Autodesk Inventor part; units mm, degrees
ref_plane "Work Plane3" through (14, 0, 0) normal (-1, 0, 0) x (0, 0, 1)
ref_plane "YZ Plane" through (0, 0, 0) normal (1, 0, 0) x (0, 1, 0)
ref_plane "XZ Plane" through (0, 0, 0) normal (0, 1, 0) x (-1, 0, 0)
sketch "Sketch1" plane through (0, 0, 0) normal (0, 0, 1) x (1, 0, 0)
  line L0 (0, 0) -> (28, 0)
  line L1 (28, 0) -> (28, 28)
  line L2 (28, 28) -> (0, 28)
  line L3 (0, 28) -> (0, 0)
  circle A0 centre (7, 0) radius 4
  circle A1 centre (21, 0) radius 4
  point P0 (3, 0)
  point P1 (11, 0)
  point P2 (17, 0)
  point P3 (25, 0)
  dimension "d0" = 28
  dimension "d1" = 28
  dimension "d2" = 8
  dimension "d3" = 8
  dimension "d4" = 14
  dimension "d5" = 7
  dimension "d6" = 7
extrude "Extrusion1" add sketch "Sketch1" along normal blind 12 contours A1 L0 A0 L3 L2 L1
chamfer "Chamfer1" distance 0.5 angle 45 4 edges at (3, 0, 6) (11, 0, 6) (17, 0, 6) (25, 0, 6)
sketch "Sketch2" plane through (0, 28, 0) normal (0, 1, 0) x (1, 0, 0)
  circle A0 centre (14, -6) radius 6.35
  line L0 (28, 0) -> (0, 0)
  line L1 (28, 0) -> (28, -12)
  point P0 (14, 0)
  point P1 (28, -6)
  point P2 (16.0791, 0)
  point P3 (11.9209, 0)
  dimension "d12" = 12.7
extrude "Extrusion2" cut sketch "Sketch2" against normal blind 4 contours A0 L0 picked at (13.6383, -8.0675)
fillet "Fillet1" radius 0.25 4 edges at (11.9209, 26, 0) (16.0791, 26, 0) (11.9209, 26, 12) (16.0791, 26, 12)
ref_plane "Work Plane3" through (14, 0, 0) normal (-1, 0, 0) x (0, 0, 1)
sketch "Sketch5" plane through (0, 0, 0) normal (0, -1, 0) x (1, 0, 0)
  circle A0 centre (-3.5, 6) radius 2
  circle A1 centre (-3.5, 6) radius 3.5
  circle A2 centre (-3.5, 6) radius 6
  line L0 (2.5, 12) -> (2.5, 0)
  line L1 (0, 12) -> (2.5, 12)
  line L2 (0, 0) -> (0, 12)
  line L3 (0, 0) -> (2.5, 0)
  line L4 (0, 0) -> (0, 12)
  line L5 (0, 0) -> (-5.9853, 0)
  line L6 (-5.9853, 0) -> (-7.7426, 1.7574)
  line L7 (0, 12) -> (-5.9853, 12)
  line L8 (-5.9853, 12) -> (-7.7426, 10.2426)
  line L9 (0, 0) -> (0, 12)
  dimension "d22" = 4
  dimension "d23" = 7
  dimension "d24" = 135
  dimension "d25" = 135
extrude "Extrusion3" add sketch "Sketch5" against normal blind 7 contours A0 | A1 | L2 A2 | L2 L5 A2 | A2 L7 L2 | L5 L6 A2 | A2 L8 L7 picked at (-7.4809, 9.2519)
sketch "Sketch6" plane through (2.5, 0, 0) normal (0, -1, 0) x (1, 0, 0)
  arc A0 (-10.2426, 10.2426) -> (-10.2426, 1.7574) centre (-6, 6) ccw
  point P0 (-2.5, 0)
hole "Hole1" at (-3.5, 0, 6) direction (0, 1, 0) diameter 4 end through all
mirror "Mirror2" about plane through (14, 0, 0) normal (-1, 0, 0) of "Extrusion3", "Hole1"
sketch "Sketch7" plane through (0, 0, 12) normal (0, 0, 1) x (1, 0, 0)
  line L0 (17.24, 24) -> (10.76, 24)
  line L1 (17.1173, 24) -> (17.24, 24)
  line L2 (17.1173, 24) -> (17.1173, 24)
  line L3 (17.24, 24) -> (17.1173, 24)
  line L4 (10.76, 24) -> (17.24, 24)
  line L5 (10.8827, 24) -> (10.76, 24)
  line L6 (10.8827, 24) -> (10.8827, 24)
  line L7 (10.76, 24) -> (10.8827, 24)
  line L8 (17.1173, 24) -> (20.35, 24)
  line L9 (7.65, 24) -> (10.8827, 24)
  line L10 (28, 28) -> (17.24, 28)
  line L11 (22.62, 28) -> (22.62, 24)
  line L12 (28, 7) -> (28, 28)
  line L13 (22.62, 24) -> (28, 7)
  line L14 (10.76, 28) -> (0, 28)
  line L15 (5.38, 28) -> (5.38, 24)
  line L16 (0, 28) -> (0, 7)
  line L17 (5.38, 24) -> (0, 7)
  line L18 (17.24, 24) -> (10.76, 24)
  point P0 (0, 0)
extrude "Extrusion4" cut sketch "Sketch7" against normal through all
chamfer "Chamfer2" distance 2 angle 45 8 edges at (22.62, 26, 12) (25.31, 15.5, 12) (22.62, 26, 0) (25.31, 15.5, 0) (2.69, 15.5, 12) (2.69, 15.5, 0) (5.38, 26, 0) (5.38, 26, 12)
equation "\"d1\" = MotorHeight"
equation "\"d5\" = d6"
equation "\"MotorHeight\" = MotorHeightBase"
properties part number "Magnet Mount"
Can you work these out from the model? Positions are in its coordinate system, mm. A direction names the side the tool comes from. Coordinates: 2 decimals unless noted, no trailing zeros. Order: outer loops, then holes, each group sorted by start corner. A loop starts at its lowest first (then second) coordinate and runs counter-clockwise, first axis right, second up. Notation, with made-up numbers: (-37, 75.5) - (1, 75.5) arc R19 ccw to (1, 111.5) - close; hole circle Ø1 at (29.25, 0.25). An arc over 180 degrees is marked (long way). Answer as a JSON object with one key per item and string values. Group by question number.
Q1. Imagine slicing it at B-B (z = 6). Give the number of separate pieces and of enclosed holes in the cut face, and give its area (3 significant figures).
Q2. We'd pull the mould along X, two halves only. Please class faces 1 (the face through (-1, 0, 6)), 2 (the face through (24.258, 15.462, 11.014)), 3 (the face through (7.65, 26.03, 5.91)): +X half, -X half, draft (parallel to the pull), parting line (faces both ways), or undercut.
Q3. Imagine slicing it at D-D (x = 15). Please give me the cut outline in (y, z), and give its area (3 significant figures).
Q4. On a 3-axis mill with a long thin cutter (end or side, diameter ignored), from which of +Z, -Z, +X, -X, +Y, -Y can I reach the whole of each face in a straight line? I mean faces 4 (the face through (6.39, 25.88, 11.01)), 5 (the face through (21.63, 25.82, 1.01)), 6 (the face through (14, 24, 6)), 7 (the face through (22.62, 26, 6)). Say none if no direction works.
Q5. Imagine slicing it at C-C (y = 13.75). Please give me the cut outline in (x, z).
Q6. Imagine slicing it at A-A (x = -3.5). Please give me the cut outline in (y, z), and give its area (3 significant figures).
Q7. I need wall thicknesses on line 1 (X direction, y = 4.25, z = 6); line 2 (X direction, y = 3.5, z = 9.5); line 3 (Z direction, x = 31.5, y = 2). Which ranges of each line are inside material? Lowest first, please. Write a range as from..to.
Q8. Will these pins go through, and if not, where does the flat tip stop? P1, Ø1, axis at x = 12.5, z = 2, coming from the -Y side; P2, Ø1, axis at x = 17.5, z = 5.5, coming from the -Y side; P3, Ø2.5, axis at x = 31.5, z = 6, coming from the +Y side; P4, Ø4, axis at y = 15, z = 8, coming from the +X side.
Determined:
{
 "1": {"separate pieces": "3", "enclosed holes": "0", "area": "625 mm2"},
 "2": {"face 1": "draft", "face 2": "+X half", "face 3": "undercut"},
 "3": {"outline": "(0, 0) - (24, 0) - (24, 12) - (0, 12) - close", "area": "288 mm2"},
 "4": {"face 4": "+Z, -X, +Y", "face 5": "-Z, +X, +Y", "face 6": "+Y", "face 7": "+Z, -Z, +X, +Y"},
 "5": {"outline": "(2.14, 2) - (4.23, 0) - (23.77, 0) - (25.86, 2) - (25.86, 10) - (23.77, 12) - (4.23, 12) - (2.14, 10) - close"},
 "6": {"outline": "(0, 0) - (7, 0) - (7, 4) - (0, 4) - close; (0, 8) - (7, 8) - (7, 12) - (0, 12) - close", "area": "56.0 mm2"},
 "7": {"line 1": "x = -9.5..-5.5, -1.5..29.5, 33.5..37.5", "line 2": "x = -8.37..5.06, 8.94..19.06, 22.94..36.37", "line 3": "z = 0..4, 8..12"},
 "8": {"P1": "stops at y = 0", "P2": "stops at y = 0.47", "P3": "passes through", "P4": "stops at x = 26.1"}
}
